For this review, take the finished solid that the model builds, in its own axes (mm). Face numbers are marked on the shaded views. A direction names the side the tool comes from. Coordinates: 2 decimals unless noted, no trailing zeros. Order: outer loops, then holes, each group sorted by start corner. A loop starts at its lowest first (then second) coordinate and runs counter-clockwise, first axis right, second up. Notation, with made-up numbers: (82.5, 73.5) -> (111.5, 73.5) arc R26 ccw to (111.5, 95.5) -> close; hole circle Ø2 at (-18, 38). An arc over 180 degrees is marked (long way). Return JSON: item names as keys, results as strings. Group by question number.
Item 1: Take a section at A-A (y = 4.5). Write out the cut boundary in (x, z).
Item 2: Machinability: for the marked faces 1, 2 and 3, which of the approach directions +Z, -Z, +X, -X, +Y, -Y give a long, thin tool a straight path to every point of the face, cutting with its end or side? Answer none if there is none.
Item 3: Take a section at D-D (x = 3.75). Write out the cut boundary in (y, z), then the cut area to 3 significant figures.
Item 4: Take a section at C-C (z = 5.75). Write out the cut boundary in (x, y).
Item 5: Draft analysis for pull direction Y (two halves, no side actions). For the marked faces 4, 5 and 6, state which applies: +Y half, -Y half, draft (parallel to the pull), parting line (faces both ways), or undercut.
Item 6: Take a section at B-B (x = 0). Write out the cut boundary in (y, z).
Item 7: Insertion check: pin 1 (2 mm diameter, centred on y = 3, z = 2.5, fed in from +X); pin 2 (3 mm diameter, centred on x = -3, z = 5.2, fed in from -Y); pin 3 (5 mm diameter, centred on y = 6.5, z = -0.5, fed in from -X). Each pin has a flat end and moves straight along its axis. Give the tip position at first contact, or say it passes through.
Item 8: For line 1 along Y through (x, z) = (0, -0.2); line 2 along Y through (x, z) = (-2.75, 7); line 3 along X through (y, z) = (7.25, 5), list the stretches that pass through material, from the lowest coordinate up.
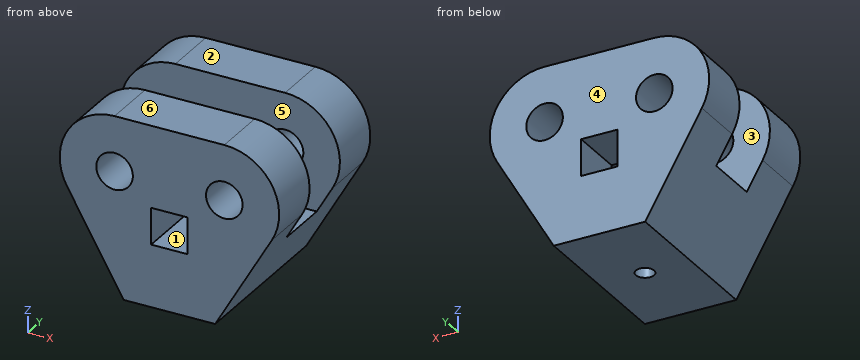
```python
from build123d import *

# Parameters (mm, degrees)
CROQUIS1_R              = 1
CROQUIS1_W              = 2
CROQUIS1_H              = 2
SALIENTE_EXTRUIR1_DEPTH = 9
CROQUIS2_W              = 12
CROQUIS2_H              = 3
CORTAR_EXTRUIR1_DEPTH   = 6
CORTAR_EXTRUIR2_REACH   = 16.64
CROQUIS3_R              = 0.5


with BuildPart() as part:
    # Croquis1 → Saliente-Extruir1 (new body)
    with BuildSketch(Plane(origin=(0, 0, 0), x_dir=(1, 0, 0), z_dir=(0, 1, 0))):
        with BuildLine():
            Line((5.598076211, -3.696152423), (2.5, 1.669872981))
            Line((2.5, 1.669872981), (-2.5, 1.669872981))
            Line((-2.5, 1.669872981), (-5.598076211, -3.696152423))
            ThreePointArc((-5.598076211, -3.696152423), (-5.598076211, -6.696152423), (-3, -8.196152423))
            Line((-3, -8.196152423), (3, -8.196152423))
            ThreePointArc((3, -8.196152423), (5.598076211, -6.696152423), (5.598076211, -3.696152423))
        make_face()
        with Locations(Location((-3, -5.196152423, 0), (0, 0, 270))):
            Circle(CROQUIS1_R, mode=Mode.SUBTRACT)
        with Locations(Location((3, -5.196152423, 0), (0, 0, 270))):
            Circle(CROQUIS1_R, mode=Mode.SUBTRACT)
        with Locations((0, -2.732050808)):
            Rectangle(CROQUIS1_W, CROQUIS1_H, mode=Mode.SUBTRACT)
    extrude(amount=SALIENTE_EXTRUIR1_DEPTH)

    # Croquis2 → Cortar-Extruir1 (cut)
    with BuildSketch(Plane.XY.offset(8.196152423)):
        with Locations((0, 4.5)):
            Rectangle(CROQUIS2_W, CROQUIS2_H)
    extrude(amount=-CORTAR_EXTRUIR1_DEPTH, mode=Mode.SUBTRACT)

    # Croquis3 → Cortar-Extruir2 (cut, up to next)
    with BuildSketch(Plane(origin=(0, 0, -1.669872981), x_dir=(-1, 0, 0), z_dir=(0, 0, -1)), mode=Mode.PRIVATE) as cortar_extruir2_sk1:
        with Locations((0, 4.5)):
            Circle(CROQUIS3_R)
    cortar_extruir2_tool1 = extrude(cortar_extruir2_sk1.sketch, amount=-CORTAR_EXTRUIR2_REACH, mode=Mode.PRIVATE) & part.part
    add(cortar_extruir2_tool1.solids().sort_by_distance((0, 4.5, -1.669873))[0], mode=Mode.SUBTRACT)


solid = part.part
```
Findings below:
{
 "1": {"outline": "(-4.73, 2.2) -> (-2.5, -1.67) -> (-0.5, -1.67) -> (-0.5, 1.73) -> (-1, 1.73) -> (-1, 2.2) -> close; (0.5, -1.67) -> (2.5, -1.67) -> (4.73, 2.2) -> (1, 2.2) -> (1, 1.73) -> (0.5, 1.73) -> close"},
 "2": {"face 1": "+Y, -Y", "face 2": "+Z, +X, -X, +Y, -Y", "face 3": "+Z, +X, -X"},
 "3": {"outline": "(0, 0.5) -> (9, 0.5) -> (9, 4.53) -> (6, 4.53) -> (6, 2.2) -> (3, 2.2) -> (3, 4.53) -> (0, 4.53) -> close; (0, 5.86) -> (3, 5.86) -> (3, 8.1) -> (0, 8.1) -> close; (6, 5.86) -> (9, 5.86) -> (9, 8.1) -> (6, 8.1) -> close", "area": "42.8 mm2"},
 "4": {"outline": "(-5.95, 0) -> (-3.83, 0) -> (-3.83, 3) -> (-5.95, 3) -> close; (-5.95, 6) -> (-3.83, 6) -> (-3.83, 9) -> (-5.95, 9) -> close; (-2.17, 0) -> (2.17, 0) -> (2.17, 3) -> (-2.17, 3) -> close; (-2.17, 6) -> (2.17, 6) -> (2.17, 9) -> (-2.17, 9) -> close; (3.83, 0) -> (5.95, 0) -> (5.95, 3) -> (3.83, 3) -> close; (3.83, 6) -> (5.95, 6) -> (5.95, 9) -> (3.83, 9) -> close"},
 "5": {"face 4": "+Y half", "face 5": "undercut", "face 6": "draft"},
 "6": {"outline": "(0, -1.67) -> (4, -1.67) -> (4, 1.73) -> (0, 1.73) -> close; (0, 3.73) -> (3, 3.73) -> (3, 8.2) -> (0, 8.2) -> close; (5, -1.67) -> (9, -1.67) -> (9, 1.73) -> (5, 1.73) -> close; (6, 3.73) -> (9, 3.73) -> (9, 8.2) -> (6, 8.2) -> close"},
 "7": {"pin 1": "stops at x = 5.48", "pin 2": "stops at y = 0", "pin 3": "stops at x = -4.62"},
 "8": {"line 1": "y = 0 to 4, 5 to 9", "line 2": "y = 0 to 3, 6 to 9", "line 3": "x = -5.99 to -3.98, -2.02 to 2.02, 3.98 to 5.99"}
}
